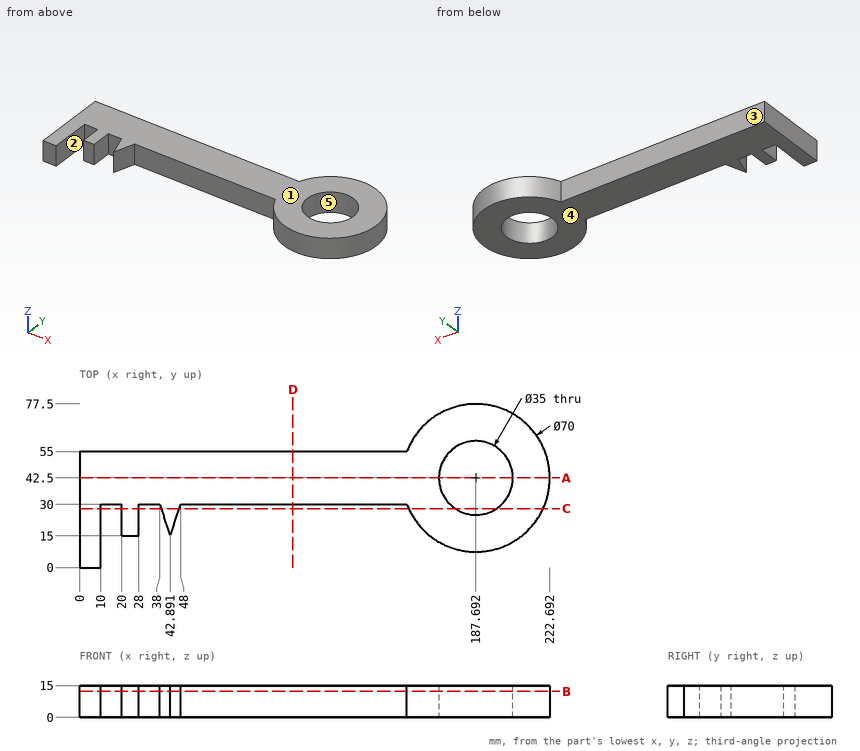
Could you check a few things on this drawing? It's one solid part, dimensions in mm from its lowest x, y, z. A direction names the side the tool comes from. Coordinates: 2 decimals unless noted, no trailing zeros. Loops run counter-clockwise (first coordinate to the right, second up) from the corner with the lowest first, then second, coordinate; pieces in that order, holes last.
1. Imagine slicing it at B-B (z = 12.25). Please give me the cut outline in (x, y), and give its area (3 significant figures).
2. For the marked faces 1, 2 and 3, which set-ups out of +Z, -Z, +X, -X, +Y, -Y let a thin tool reach every point of the face, with its end or its side?
3. Imagine slicing it at A-A (y = 42.5). Please give me the cut outline in (x, z), and give its area (3 significant figures).
4. I need wall thicknesses on L1, parallel to X at y = 29.5, z = 12 (1 decimal); L2, parallel to X at y = 21, z = 6.75 (1 decimal); L3, parallel to Y at x = 68, z = 4. Which ranges of each line are inside material? Lowest first, please.
5. For P1, Ø7.5, axis at y = 20, z = 10, coming from the +X side (1 decimal); P2, Ø1.5, axis at x = 29.5, z = 10.5, coming from the +Y side; P3, Ø6, axis at y = 46.5, z = 9.5, coming from the +X side, each with a flat end and sliding along its axis, tell me the tip position at first contact or that it passes through.
6. Imagine slicing it at D-D (x = 101). Please give me the cut outline in (y, z), and give its area (3 significant figures).
7. Imagine slicing it at C-C (y = 28). Please give me the cut outline in (x, z), and give its area (3 significant figures).
8. We'd pull the mould along X, two halves only. Please class the marked faces 4 and 5: released by +X, released by -X, zero draft, split by the parting line, or undercut.
Computed values:
1. outline: (0, 0) - (10, 0) - (10, 30) - (20, 30) - (20, 15) - (28, 15) - (28, 30) - (38, 30) - (42.89, 15) - (48, 30) - (155, 30) arc R35 ccw (long way) to (155, 55) - (0, 55) - close; hole circle Ø35 at (187.69, 42.5)
1. area: 7,220 mm2
2. face 1: +Z, +X, -X, +Y, -Y
2. face 2: +Z, -Z, -Y
2. face 3: +Z, -Z, -X, +Y
3. outline: (0, 0) - (170.19, 0) - (170.19, 15) - (0, 15) - close; (205.19, 0) - (222.69, 0) - (222.69, 15) - (205.19, 15) - close
3. area: 2,820 mm2
4. L1: x = 0 to 10, 20 to 28, 38.2 to 47.8, 155.2 to 176, 199.4 to 220.2
4. L2: x = 0 to 10, 20 to 28, 40.9 to 44.9, 160.1 to 215.3
4. L3: y = 30 to 55
5. P1: stops at x = 217.2
5. P2: stops at y = 55
5. P3: stops at x = 222.68
6. outline: (30, 0) - (55, 0) - (55, 15) - (30, 15) - close
6. area: 375 mm2
7. outline: (0, 0) - (10, 0) - (10, 15) - (0, 15) - close; (20, 0) - (28, 0) - (28, 15) - (20, 15) - close; (38.65, 0) - (47.32, 0) - (47.32, 15) - (38.65, 15) - close; (155.84, 0) - (177.89, 0) - (177.89, 15) - (155.84, 15) - close; (197.49, 0) - (219.55, 0) - (219.55, 15) - (197.49, 15) - close
7. area: 1,060 mm2
8. face 4: zero draft
8. face 5: undercut
